```python
from build123d import *

# Parameters (mm, degrees)
SKETCH_1_W      = 26.5
SKETCH_1_H      = 54.6
EXTRUDE_1_DEPTH = 1.5
SKETCH_3_W      = 9.37884322
SKETCH_3_H      = 1.093530985
EXTRUDE_2_DEPTH = 3
SKETCH_4_W      = 9.519823585
SKETCH_4_H      = 4.812938029
SKETCH_4_W_2    = 7.971209668
SKETCH_4_H_2    = 13
EXTRUDE_3_DEPTH = 3.5


with BuildPart() as part:
    # ｽｹｯﾁ1 → ﾎﾞｽ - 押し出し1 (new body)
    with BuildSketch(Plane.XY):
        with Locations((29.00738196, 33.991909398)):
            Rectangle(SKETCH_1_W, SKETCH_1_H)
    extrude(amount=EXTRUDE_1_DEPTH)

    # ｽｹｯﾁ3 → ﾎﾞｽ - 押し出し2 (add)
    with BuildSketch(Plane(origin=(0, 0, 0), x_dir=(-1, 0, 0), z_dir=(0, 0, -1))):
        with Locations((-37.56796035, 60.745143906)):
            Rectangle(SKETCH_3_W, SKETCH_3_H)
    extrude_2 = extrude(amount=EXTRUDE_2_DEPTH)

    # ﾐﾗｰ1: ﾎﾞｽ - 押し出し2 across plane
    add(extrude_2.mirror(Plane(origin=(0, 33.991909398, 0), x_dir=(0, 0, 1), z_dir=(0, -1, 0))))

    # ｽｹｯﾁ4 → ﾎﾞｽ - 押し出し3 (add)
    with BuildSketch(Plane(origin=(0, 0, 0), x_dir=(-1, 0, 0), z_dir=(0, 0, -1))):
        with Locations((-37.497470167, 33.991909398)):
            Rectangle(SKETCH_4_W, SKETCH_4_H)
        with Locations((-19.742986794, 33.991909398)):
            Rectangle(SKETCH_4_W_2, SKETCH_4_H_2)
    extrude(amount=EXTRUDE_3_DEPTH)


solid = part.part
```
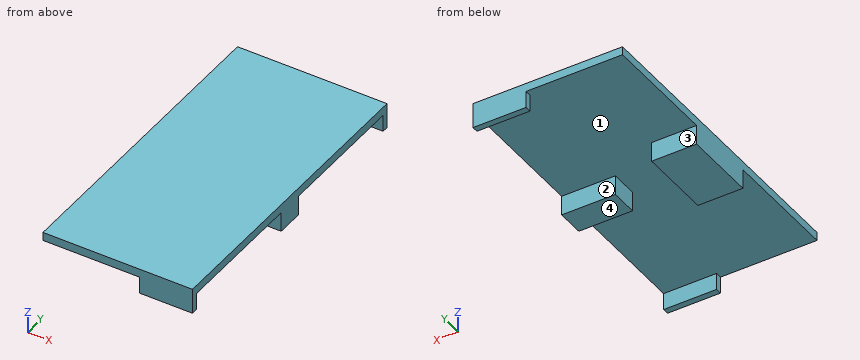
Geometry check sheet. Reference: the model listing, model coordinates, mm. Face numbers are marked on the shaded views. Round coordinates to 2 decimals unless told otherwise and drop trailing zeros. Loops run counter-clockwise (first coordinate to the right, second up) from the corner with the lowest first, then second, coordinate; pieces in that order, holes last. Notation, with made-up numbers: (70, -7) - (104, -7) arc R28 cw to (104, 32) - close; hole circle Ø2 at (89.5, 22.25). An arc over 180 degrees is marked (long way). Write item = value, one per line. Start each with the question number.
1. Section check D-D on x = 19. Enter the section's corners in (y, z), then the cut area to 3 significant figures.
2. Mould release check, pull along Y, two halves, no side actions. Record for the marked faces 1, 2, 3 and 4: released by +Y, released by -Y, zero draft, split by the parting line, or undercut.
3. Depth check by flat-ended pin: pin 1 (6 mm diameter, centred on x = 31.5, y = 21.5, fed in from -Z); pin 2 (0.9 mm diameter, centred on y = 7.5, z = -2, fed in from -X); pin 3 (1.2 mm diameter, centred on x = 39.5, y = 60.5, fed in from -Z). Enter the tip coordinate at first touch or a pass-through.
4. Thickness scan on line 1 (Y direction, x = 37, z = -1.05); line 2 (Z direction, x = 33, y = 17.5); line 3 (X direction, y = 29.5, z = -0.55). Record the ranges inside material, lowest first.
5. Section check B-B on x = 37. Enter the section's corners in (y, z), then the cut area to 3 significant figures.
6. Section check A-A on z = -0.55. Enter the section's corners in (x, y).
7. Section check C-C on y = 14. Enter the section's corners in (x, z), then the cut area to 4 significant figures.
Working result:
q1.outline = (6.69, 0) - (27.49, 0) - (27.49, -3.5) - (40.49, -3.5) - (40.49, 0) - (61.29, 0) - (61.29, 1.5) - (6.69, 1.5) - close
q1.area = 127 mm^2
q2.face_1 = undercut
q2.face_2 = undercut
q2.face_3 = released by +Y
q2.face_4 = zero draft
q3.pin_1 = 0
q3.pin_2 = 32.88
q3.pin_3 = -3
q4.line_1 = 6.69 to 7.79, 31.59 to 36.4, 60.2 to 61.29
q4.line_2 = 0 to 1.5
q4.line_3 = 15.76 to 23.73
q5.outline = (6.69, -3) - (7.79, -3) - (7.79, 0) - (31.59, 0) - (31.59, -3.5) - (36.4, -3.5) - (36.4, 0) - (60.2, 0) - (60.2, -3) - (61.29, -3) - (61.29, 1.5) - (6.69, 1.5) - close
q5.area = 105 mm^2
q6.outline = (15.76, 27.49) - (23.73, 27.49) - (23.73, 40.49) - (15.76, 40.49) - close; (32.74, 31.59) - (42.26, 31.59) - (42.26, 36.4) - (32.74, 36.4) - close; (32.88, 6.69) - (42.26, 6.69) - (42.26, 7.79) - (32.88, 7.79) - close; (32.88, 60.2) - (42.26, 60.2) - (42.26, 61.29) - (32.88, 61.29) - close
q7.outline = (15.76, 0) - (42.26, 0) - (42.26, 1.5) - (15.76, 1.5) - close
q7.area = 39.75 mm^2
